```python
from build123d import *


# Read off the part's stored shape, not the designer's step: M5 机械螺纹 螺柱1
with BuildPart() as part:
    # 草图1 → 旋转1 (revolve)
    with BuildSketch(Plane.XY, mode=Mode.PRIVATE) as revolve_1_sk:
        Polygon((0, 0), (0, 24.25), (4.5, 24.25), (4.5, 19.75), (3, 19.75), (3, 9.75), (2.8, 9.75), (2.8, 0), align=None)
    revolve(revolve_1_sk.sketch.rotate(Axis((0, 0, 0), (0, 1, 0)), 90), axis=Axis((0, 0, 0), (0, 1, 0)))

    # M5 机械螺纹 螺柱1 outline → M5 机械螺纹 螺柱1 (revolve, cut)
    with BuildSketch(Plane.XY):
        Polygon((2.8, 9.75), (2.5, 9.75), (2.5, 0.433), (2.067, 0), (2.8, 0), align=None)
    revolve(axis=Axis((0, 0, 0), (0, 1, 0)), mode=Mode.SUBTRACT)


solid = part.part
```
CAD build for the part. Positions are in the model's coordinates, mm. A direction names the side the tool comes from. Round coordinates to 2 decimals unless told otherwise and drop trailing zeros. Write each loop counter-clockwise with the first axis right and the second up, starting at its lowest first coordinate (ties: lowest second). Pieces come first, ordered by that corner, then holes. Notation, with made-up numbers: (-23.75, -11.5) -> (23.25, -11.5) arc R19 cw to (23.25, 25.5) -> close; hole circle Ø5 at (-19, 16.5). An arc over 180 degrees is marked (long way). Answer in a Markdown table with one row per item. Add a question column.
Item 1: Saw through at B-B, the plane z = 0. Write the cut outline in (x, y), then the cut area to 3 significant figures.
Item 2: Saw through at A-A, the plane x = 0. Write the cut outline in (y, z).
Item 3: Drill centre lines: line 1 (Y direction, x = -0.5, z = -3.75); line 2 (Y direction, x = -2.5, z = 1.25); line 3 (X direction, y = 10, z = -2.75). Where is each one in solid material? Low to high. Write a range as from..to.
Item 4: Which spindle directions (+Z, -Z, +X, -X, +Y, -Y) get a long thin tool onto all of the face, cutting with end or side? Do faces 1 (the face through (-2, 9.75, 2)), 2 (the face through (-3.04, 21.97, 3.32)). Say none if no direction does.
Item 5: Saw through at D-D, the plane y = 18.25. Write the cut outline in (x, z).
Item 6: Drop flat-ended pins along their axis: pin 1 Ø1.5 at (y, z) = (16, -0.5) entering from -X; pin 2 Ø1 at (x, y) = (-1, 10) entering from -Z; pin 3 Ø4 at (y, z) = (20.5, 3.5) entering from +X. Give the stop position or say it passes through.
Item 7: Saw through at C-C, the plane y = 5.25. Write the cut outline in (x, z), then the cut area to 3 significant figures.
Findings below:
| question | item | result |
|---|---|---|
| 1 | outline | (-4.5, 19.75) -> (-3, 19.75) -> (-3, 9.75) -> (-2.5, 9.75) -> (-2.5, 0.43) -> (-2.07, 0) -> (2.07, 0) -> (2.5, 0.43) -> (2.5, 9.75) -> (3, 9.75) -> (3, 19.75) -> (4.5, 19.75) -> (4.5, 24.25) -> (-4.5, 24.25) -> close |
| 1 | area | 149 mm^2 |
| 2 | outline | (0, -2.07) -> (0.43, -2.5) -> (9.75, -2.5) -> (9.75, -3) -> (19.75, -3) -> (19.75, -4.5) -> (24.25, -4.5) -> (24.25, 4.5) -> (19.75, 4.5) -> (19.75, 3) -> (9.75, 3) -> (9.75, 2.5) -> (0.43, 2.5) -> (0, 2.07) -> close |
| 3 | line 1 | y = 19.75..24.25 |
| 3 | line 2 | y = 9.75..24.25 |
| 3 | line 3 | x = -1.2..1.2 |
| 4 | face 1 | -Y |
| 4 | face 2 | +Y, -Y |
| 5 | outline | circle Ø6 at (0, 0) |
| 6 | pin 1 | stops at x = -3 |
| 6 | pin 2 | stops at z = -2.96 |
| 6 | pin 3 | stops at x = 4.24 |
| 7 | outline | circle Ø5 at (0, 0) |
| 7 | area | 19.6 mm^2 |
